Check sheet for the modelled part. Datum: model origin and axes. Units: mm. Face numbers are marked on the shaded views. A direction names the side the tool comes from. Give positions to 0.01 mm unless a question says otherwise; leave off trailing zeros. Loops run counter-clockwise (first coordinate to the right, second up) from the corner with the lowest first, then second, coordinate; pieces in that order, holes last. Notation, with made-up numbers: M -35.75,-20.75 L 1.25,-20.75 A13 cw 1.25,0.25 Z; hole C 61.25,85 d3. An arc over 180 degrees is marked long. Use one line per item in the form item = value.
from build123d import *

# Parameters (mm, degrees)
SKETCH1_W           = 35.1
SKETCH1_H           = 35.1
BOSS_EXTRUDE1_DEPTH = 29
SKETCH2_R           = 11.25
BOSS_EXTRUDE2_DEPTH = 2.5
SKETCH3_R           = 2.75
BOSS_EXTRUDE3_DEPTH = 20


with BuildPart() as part:
    # Sketch1 → Boss-Extrude1 (new body)
    with BuildSketch(Plane.XY):
        with Locations((4.3875, -9)):
            Rectangle(SKETCH1_W, SKETCH1_H)
    extrude(amount=BOSS_EXTRUDE1_DEPTH)

    # Sketch2 → Boss-Extrude2 (add)
    with BuildSketch(Plane.XY.offset(29)):
        with Locations((4.3875, -9)):
            Circle(SKETCH2_R)
    extrude(amount=BOSS_EXTRUDE2_DEPTH)

    # Sketch3 → Boss-Extrude3 (add)
    with BuildSketch(Plane.XY.offset(31.5)):
        with Locations((4.3875, -9)):
            Circle(SKETCH3_R)
    extrude(amount=BOSS_EXTRUDE3_DEPTH)


solid = part.part
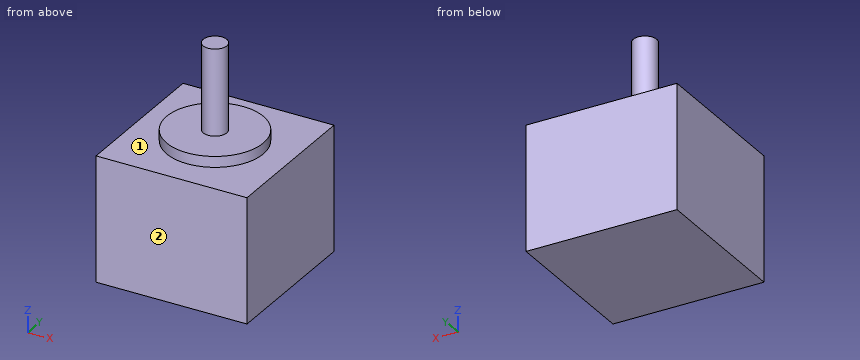
1) Set-up check for the marked faces 1 and 2: record each of +Z, -Z, +X, -X, +Y, -Y from which the full face is reachable in a straight line by a thin tool's end or side.
Evaluation:
face_1 = +Z
face_2 = +Z, -Z, +X, -X, -Y
2) Section check C-C (z = 41). Record the cut outline in (x, y).
Evaluation:
outline = C 4.39,-9 d5.5
3) Section check D-D (y = 0.5). Record the cut outline in (x, z), then the cut area to 3 significant figures.
Evaluation:
outline = M -13.16,0 L 21.94,0 L 21.94,29 L 10.41,29 L 10.41,31.5 L -1.64,31.5 L -1.64,29 L -13.16,29 Z
area = 1,050 mm^2
4) Scan lines: line 1 (Z direction, x = 13.5, y = 7); line 2 (Z direction, x = 11, y = -17); line 3 (Y direction, x = 3, z = 47.5). Record each from-to range of solid material in increasing order.
Evaluation:
line_1 = 0 to 29
line_2 = 0 to 31.5
line_3 = -11.37 to -6.63
5) Section check B-B (x = 10.5). Record the cut outline in (y, z), then the cut area to 3 significant figures.
Evaluation:
outline = M -26.55,0 L 8.55,0 L 8.55,29 L 0.44,29 L 0.44,31.5 L -18.44,31.5 L -18.44,29 L -26.55,29 Z
area = 1,070 mm^2
6) Depth check by flat-ended pin: pin 1 Ø1.5 at (x, y) = (7.5, -11.5) entering from -Z; pin 2 Ø12 at (y, z) = (3, 40.5) entering from -X; pin 3 Ø10 at (y, z) = (-3, 42) entering from +X; pin 4 Ø1 at (x, y) = (-9, -11) entering from +Z. Enter the tip coordinate at first touch or a pass-through.
Evaluation:
pin_1 = 0
pin_2 = through
pin_3 = 6.95
pin_4 = 29
7) Section check A-A (y = -9). Record the cut outline in (x, z).
Evaluation:
outline = M -13.16,0 L 21.94,0 L 21.94,29 L 15.64,29 L 15.64,31.5 L 7.14,31.5 L 7.14,51.5 L 1.64,51.5 L 1.64,31.5 L -6.86,31.5 L -6.86,29 L -13.16,29 Z
